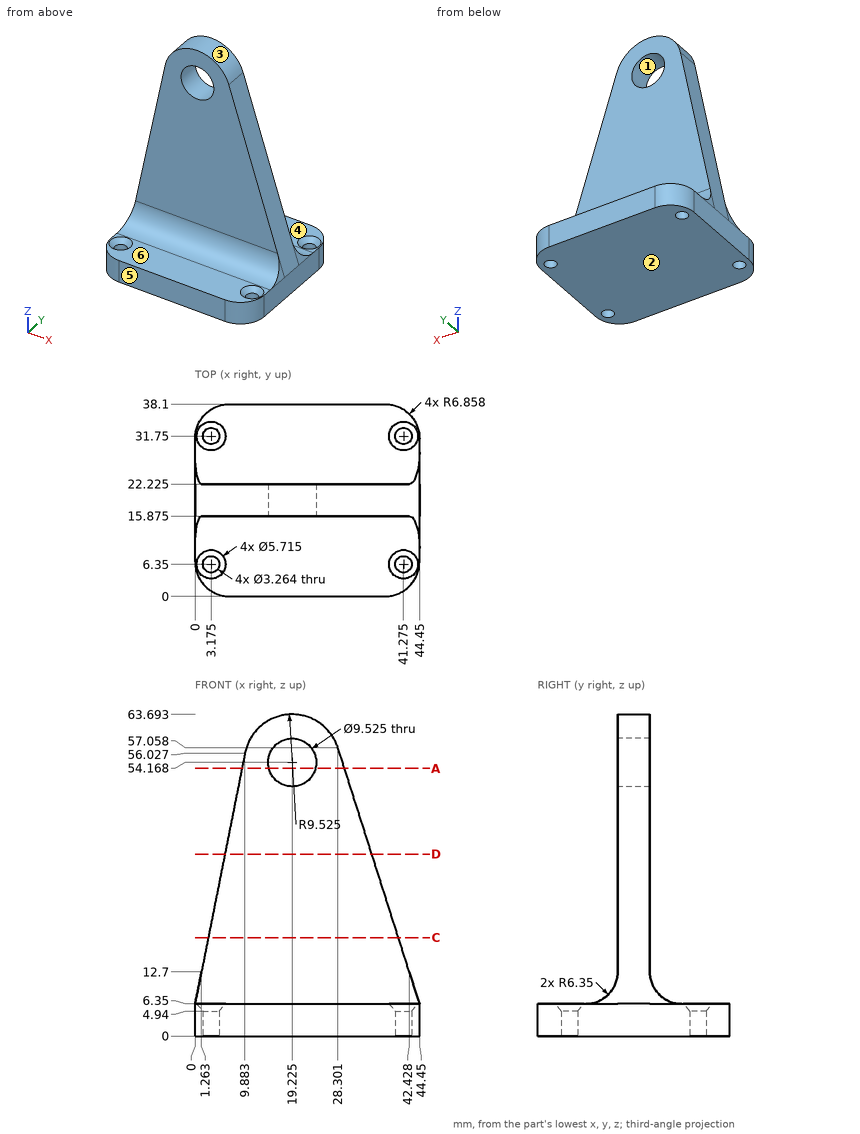
Part print with two shaded views. Sizes in mm from the minimum x, y, z corner. A direction names the side the tool comes from. Round coordinates to 2 decimals unless told otherwise and drop trailing zeros. Loops run counter-clockwise (first coordinate to the right, second up) from the corner with the lowest first, then second, coordinate; pieces in that order, holes last. Notation, with made-up numbers: M -36,44.25 L 17,44.25 A20 cw 17,79.25 Z; hole C 70,-21.5 d6. An arc over 180 degrees is marked long. Put each result on its own line as item: value. Start each with the question number.
Item 1: Drop flat-ended pins along their axis: P1, Ø4, axis at x = 27, z = 55, coming from the -Y side (3 decimals); P2, Ø10, axis at x = 27, z = 16, coming from the +Y side; P3, Ø2, axis at x = 38.5, y = 7, coming from the +Z side. Give the stop position or say it passes through.
Item 2: Mould opens along X. For the marked faces 1, 2 and 3 say: released by +X, released by -X, zero draft, split by the parting line, or undercut.
Item 3: 3-axis set-ups, long thin cutter, end or side, ignore diameter. For the marked faces 4, 5 and 6: which of +Z, -Z, +X, -X, +Y, -Y reach the whole face in a straight line?
Item 4: Drill centre lines: line 1 along Z through (x, y) = (19, 20.5) (1 decimal); line 2 along Y through (x, z) = (30, 25.5) (1 decimal); line 3 along Z through (x, y) = (35, 3). Where is each one in solid material? Low to high.
Item 5: Cut at A-A (z = 53). List the corners of the cut face in (x, y) (1 decimal).
Item 6: Cut at D-D (z = 36). List the corners of the cut face in (x, y) (1 decimal), then the cut area to 3 significant figures.
Item 7: Cut at C-C (z = 19.5). List the corners of the cut face in (x, y) (1 decimal).
Answer block:
1. P1: y = 15.875
1. P2: y = 22.46
1. P3: z = 6.35
2. face 1: undercut
2. face 2: zero draft
2. face 3: split by the parting line
3. face 4: +Z, +X, -X, +Y
3. face 5: +Z, -Z, +X, -X, -Y
3. face 6: +Z, +X, -X, -Y
4. line 1: 0 to 49.4, 58.9 to 63.7
4. line 2: 15.9 to 22.2
4. line 3: 0 to 6.35
5. outline: M 9.3,15.9 L 14.6,15.9 L 14.6,22.2 L 9.3,22.2 Z; M 23.8,15.9 L 29.6,15.9 L 29.6,22.2 L 23.8,22.2 Z
6. outline: M 5.9,15.9 L 35,15.9 L 35,22.2 L 5.9,22.2 Z
6. area: 185 mm2
7. outline: M 2.6,15.9 L 40.3,15.9 L 40.3,22.2 L 2.6,22.2 Z
